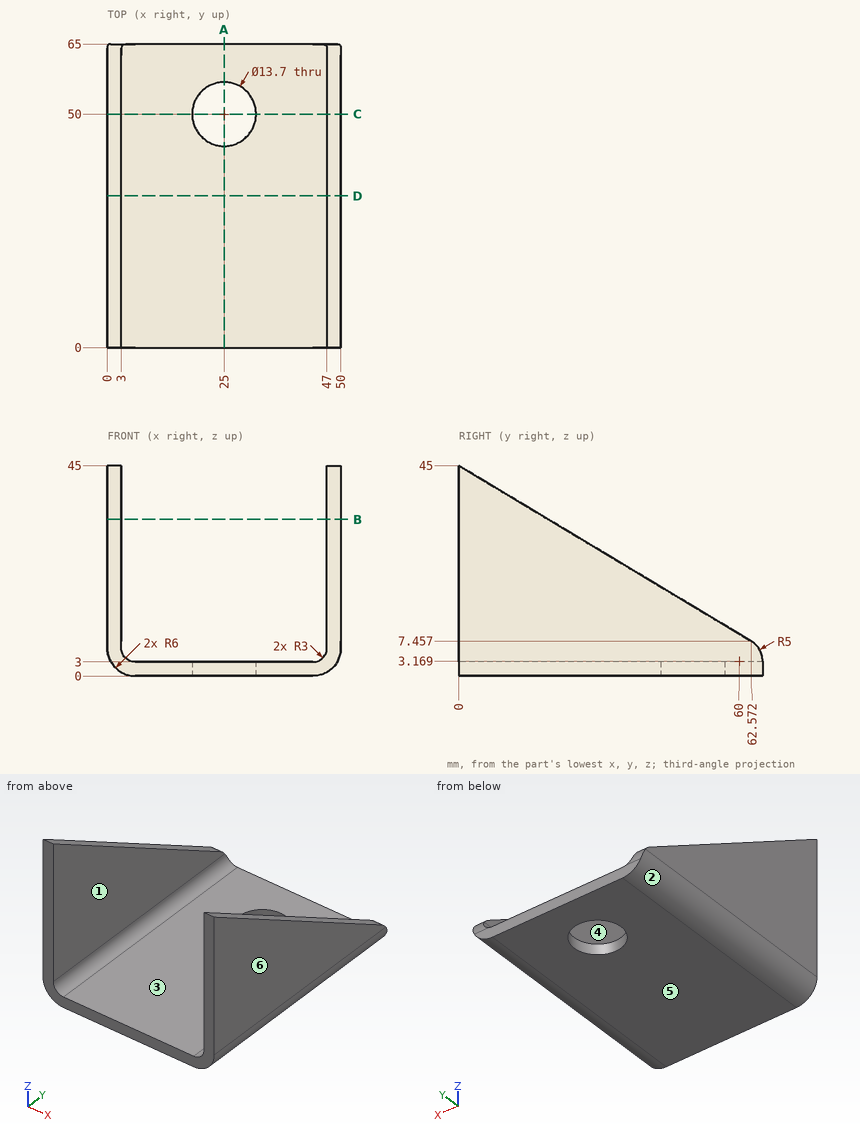
Geometry: see drawing. Coordinates: mm, zero at the bounding-box minimum. A direction names the side the tool comes from. Coordinates: 2 decimals unless noted, no trailing zeros. Order: outer loops, then holes, each group sorted by start corner. A loop starts at its lowest first (then second) coordinate and runs counter-clockwise, first axis right, second up. Notation, with made-up numbers: (62, 37) -> (66, 37) arc R21 cw to (66, 55) -> close; hole circle Ø4 at (46, 58.25). An arc over 180 degrees is marked (long way). Write each question's results on one line, items separated by ' | '. Start each with the question number.
1) Material intervals for line 1 along X through (y, z) = (27, 10.5); line 2 along Y through (x, z) = (25, 1.6); line 3 along Z through (x, y) = (10.5, 59.5), sorted ascending.
2) Cut plane D-D, the plane y = 32.5. Output: boundary loops of the cut face in (x, z).
3) Mould query, pull axis X, two halves, no side actions, for the marked faces 3, 4, 5 and 6. Classes: released by +X, released by -X, zero draft, split by the parting line, or undercut.
4) Cut plane A-A, the plane x = 25. Output: boundary loops of the cut face in (y, z).
5) Cut plane B-B, the plane z = 33.5. Output: boundary loops of the cut face in (x, y), and give its area (3 significant figures).
6) First-contact query: pin 1 (8 mm diameter, centred on x = 20.5, y = 26, fed in from +Z); pin 2 (12 mm diameter, centred on x = 37.5, z = 9.5, fed in from +Y); pin 3 (8 mm diameter, centred on y = 50, z = 18.5, fed in from +X). Flat tips, straight axial feed; report the tip coordinate or a pass-through.
7) Set-up query: the marked faces 1 and 2. Return all of +Z, -Z, +X, -X, +Y, -Y with unobstructed straight access to the full face (end or side cutting, diameter ignored); none if empty.
8) Cut plane C-C, the plane y = 50. Output: boundary loops of the cut face in (x, z).
Checks:
1) line 1: 0 to 3, 47 to 50 | line 2: 0 to 43.15, 56.85 to 65 | line 3: 0 to 3
2) outline: (0, 6) arc R6 ccw to (6, 0) -> (44, 0) arc R6 ccw to (50, 6) -> (50, 25.5) -> (47, 25.5) -> (47, 6) arc R3 cw to (44, 3) -> (6, 3) arc R3 cw to (3, 6) -> (3, 25.5) -> (0, 25.5) -> close
3) face 3: undercut | face 4: undercut | face 5: zero draft | face 6: released by +X
4) outline: (0, 0) -> (43.15, 0) -> (43.15, 3) -> (0, 3) -> close; (56.85, 0) -> (65, 0) -> (65, 3) -> (56.85, 3) -> close
5) outline: (0, 0) -> (3, 0) -> (3, 19.17) -> (0, 19.17) -> close; (47, 0) -> (50, 0) -> (50, 19.17) -> (47, 19.17) -> close | area: 115 mm^2
6) pin 1: z = 3 | pin 2: through | pin 3: x = 50
7) face 1: +Z, +Y, -Y | face 2: -Z, -X, +Y, -Y
8) outline: (0, 6) arc R6 ccw to (6, 0) -> (18.15, 0) -> (18.15, 3) -> (6, 3) arc R3 cw to (3, 6) -> (3, 15) -> (0, 15) -> close; (31.85, 0) -> (44, 0) arc R6 ccw to (50, 6) -> (50, 15) -> (47, 15) -> (47, 6) arc R3 cw to (44, 3) -> (31.85, 3) -> close
